```python
from build123d import *

# Parameters (mm, degrees)
SKETCH2_R      = 3.175
EXTRUDE1_DEPTH = 9.525
SKETCH3_W      = 25.4
SKETCH3_H      = 25.4
SKETCH3_R      = 3.175
EXTRUDE2_DEPTH = 6.35
SKETCH4_R      = 5.207
EXTRUDE3_DEPTH = 12.7
FILLET1_R      = 2


with BuildPart() as part:
    # Sketch2 → Extrude1 (new body)
    with BuildSketch(Plane.XY):
        Polygon((0, 0), (50.8, 0), (50.8, 47.625), (63.5, 47.625), (63.5, 73.025), (50.8, 73.025), (0, 73.025), align=None)
        with Locations((12.7, 60.325)):
            Circle(SKETCH2_R, mode=Mode.SUBTRACT)
        with Locations((38.1, 60.325)):
            Circle(SKETCH2_R, mode=Mode.SUBTRACT)
        Polygon((31.815804866, 18.25625), (28.607902433, 23.8125), (22.192097567, 23.8125), (18.984195134, 18.25625), (22.192097567, 12.7), (28.607902433, 12.7), align=None, mode=Mode.SUBTRACT)
    extrude(amount=EXTRUDE1_DEPTH)

    # Sketch3 → Extrude2 (add)
    with BuildSketch(Plane(origin=(63.5, 0, 0), x_dir=(0, 0, -1), z_dir=(1, 0, 0))):
        with Locations((3.175, 60.325)):
            Rectangle(SKETCH3_W, SKETCH3_H)
        with Locations((3.175, 60.325)):
            Circle(SKETCH3_R, mode=Mode.SUBTRACT)
    extrude(amount=EXTRUDE2_DEPTH)

    # Sketch4 → Extrude3 (cut)
    with BuildSketch(Plane.ZY.offset(-63.5)):
        with Locations((-3.175, 60.325)):
            Circle(SKETCH4_R)
    extrude(amount=EXTRUDE3_DEPTH, mode=Mode.SUBTRACT)

    # Fillet1
    fillet1_edges = [part.edges().sort_by_distance(p)[0] for p in [
        (50.8, 60.325, 0),
    ]]
    fillet(fillet1_edges, radius=FILLET1_R)


solid = part.part
```
Verification items for the finished model (mm, model axes). A direction names the side the tool comes from. Round coordinates to 2 decimals unless told otherwise and drop trailing zeros. Write each loop counter-clockwise with the first axis right and the second up, starting at its lowest first coordinate (ties: lowest second). Pieces come first, ordered by that corner, then holes.
1. Scan lines: L1, parallel to Y at x = 12.7, z = 3 (3 decimals); L2, parallel to X at y = 61, z = 1.75; L3, parallel to Z at x = 33.5, y = 37 (3 decimals). Record each from-to range of solid material in increasing order.
2. Draft check along X on faces 1 (the flat face through (24, 37, 0)), 2 (the cylindrical face through (57.89, 60.26, 2.03)), 3 (the cylindrical face through (37.687, 63.473, 4.696)), 4 (the flat face through (50.8, 23, 5)). Enter one of: +X half, -X half, draft (parallel to the pull), parting line (faces both ways), or undercut.
3. Section check B-B on y = 22. Enter the section's corners in (x, z) (3 decimals).
4. Section check C-C on z = 4.25. State how many separate pieces and enclosed holes the cut face has, plus the area to 3 significant figures.
5. Section check A-A on x = 12.7. Enter the section's corners in (y, z) (3 decimals).
6. Gauge pin test, flat ends, axial feed: P1, Ø3, axis at y = 13.5, z = 4.5, coming from the +X side; P2, Ø1, axis at x = 15.5, y = 30.5, coming from the -Z side; P3, Ø1.5, axis at y = 29, z = -2, coming from the -X side; P4, Ø9, axis at y = 57.5, z = -9.5, coming from the -X side. Record the tip position at first contact, or that the pin passes through.
7. Access from +Z, -Z, +X, -X, +Y, -Y to the whole of each face (thin tool, end or side, straight path). Record for faces 5 (the cylindrical face through (49.93, 60.27, 0.35)), 6 (the flat face through (69.85, 58, 0)), 7 (the flat face through (64, 47.625, 0)), 8 (the flat face through (20.566, 15.517, 4.696)).
Answer:
1. L1: y = 0 to 57.15, 63.5 to 73.025
1. L2: x = 0 to 9.6, 15.8 to 35, 41.2 to 50.78, 63.5 to 69.85
1. L3: z = 0 to 9.525
2. face 1: draft
2. face 2: undercut
2. face 3: undercut
2. face 4: +X half
3. outline: (0, 0) - (21.146, 0) - (21.146, 9.525) - (0, 9.525) - close; (29.654, 0) - (50.8, 0) - (50.8, 9.525) - (29.654, 9.525) - close
4. separate pieces: 1
4. enclosed holes: 3
4. area: 4,020 mm2
5. outline: (0, 0) - (57.15, 0) - (57.15, 9.525) - (0, 9.525) - close; (63.5, 0) - (73.025, 0) - (73.025, 9.525) - (63.5, 9.525) - close
6. P1: stops at x = 50.8
6. P2: stops at z = 0
6. P3: passes through
6. P4: stops at x = 63.5
7. face 5: -Z
7. face 6: +Z, -Z, +X, +Y, -Y
7. face 7: +Z, -Z, +X, -Y
7. face 8: +Z, -Z
